from build123d import *
from build123d.topology import SkipClean

# Parameters (mm, degrees)
SKETCH1_W           = 9
SKETCH1_H           = 9
BOSS_EXTRUDE1_DEPTH = 20
SKETCH2_W           = 6
SKETCH2_H           = 6
CUT_EXTRUDE1_DEPTH  = 21.988091862
SKETCH4_W           = 20
SKETCH4_H           = 20
BOSS_EXTRUDE2_DEPTH = 1.5
SKETCH5_W           = 20
SKETCH5_H           = 20
BOSS_EXTRUDE3_DEPTH = 3.5
SKETCH7_W           = 1.8
SKETCH7_H           = 20
CUT_EXTRUDE5_DEPTH  = 16
CUT_EXTRUDE6_START  = -1.7
CUT_EXTRUDE6_DEPTH  = 1.7
BOSS_EXTRUDE4_START = 0.5
BOSS_EXTRUDE4_DEPTH = 0.5
SKETCH10_W          = 6.2
SKETCH10_H          = 6.2
CUT_EXTRUDE8_DEPTH  = 24.748684208


with BuildPart() as part:
    # Sketch1 → Boss-Extrude1 (new body)
    with BuildSketch(Plane.XY):
        Rectangle(SKETCH1_W, SKETCH1_H)
    extrude(amount=BOSS_EXTRUDE1_DEPTH)

    # Sketch2 → Cut-Extrude1 (cut, through all)
    with BuildSketch(Plane(origin=(0, 0, 0), x_dir=(-1, 0, 0), z_dir=(0, 0, -1))):
        Rectangle(SKETCH2_W, SKETCH2_H)
    extrude(amount=-CUT_EXTRUDE1_DEPTH, mode=Mode.SUBTRACT)

    # Sketch4 → Boss-Extrude2 (add)
    with BuildSketch(Plane(origin=(4.5, 0, 0), x_dir=(0, 0, -1), z_dir=(1, 0, 0))):
        with Locations((-10, 0)):
            Rectangle(SKETCH4_W, SKETCH4_H)
    extrude(amount=-BOSS_EXTRUDE2_DEPTH)

    # Sketch5 → Boss-Extrude3 (add)
    with BuildSketch(Plane(origin=(4.5, 0, 0), x_dir=(0, 0, -1), z_dir=(1, 0, 0))):
        with Locations((-10, 0)):
            Rectangle(SKETCH5_W, SKETCH5_H)
    extrude(amount=BOSS_EXTRUDE3_DEPTH)

    # Sketch6 → Cut-Revolve2 (revolve, cut)
    with BuildSketch(Plane(origin=(0, 0, 10), x_dir=(-1, 0, 0), z_dir=(0, 0, -1)), mode=Mode.PRIVATE) as cut_revolve2_sk:
        with BuildLine():
            Line((-4.5, 7.5), (-4.5, 0))
            Line((-4.5, 0), (-7.200284, 0))
            ThreePointArc((-7.200284, 0), (-6.974408022, 3.776920415), (-6.3, 7.5))
            Line((-6.3, 7.5), (-4.5, 7.5))
        make_face()
    revolve(cut_revolve2_sk.sketch.rotate(Axis((88.99, 0, 10), (-1, 0, 0)), 90), axis=Axis((88.99, 0, 10), (-1, 0, 0)), mode=Mode.SUBTRACT)

    # Sketch7 → Cut-Extrude5 (cut)
    with BuildSketch(Plane.XZ.offset(10)):
        with Locations((5.4, 10)):
            Rectangle(SKETCH7_W, SKETCH7_H)
    extrude(amount=-CUT_EXTRUDE5_DEPTH, mode=Mode.SUBTRACT)

    # Sketch8 → Cut-Extrude6 (cut)
    with BuildSketch(Plane(origin=(8, 0, 0), x_dir=(0, 0, -1), z_dir=(1, 0, 0)).offset(CUT_EXTRUDE6_START)):
        with BuildLine():
            Line((-6.875, 0), (-6.875, -10))
            ThreePointArc((-6.875, -10), (-10, -13.125), (-13.125, -10))
            Line((-13.125, -10), (-13.125, 0))
            ThreePointArc((-13.125, 0), (-10, 3.125), (-6.875, 0))
        make_face()
    extrude(amount=CUT_EXTRUDE6_DEPTH, mode=Mode.SUBTRACT)

    # Sketch9 → Boss-Extrude4 (add)
    with SkipClean():  # the faces are left unmerged after this step: merging them gives an invalid solid
        with BuildSketch(Plane.ZY.offset(-6.3).offset(BOSS_EXTRUDE4_START)):
            with BuildLine():
                Line((13.125, -6.817945072), (13.125, -10))
                Line((13.125, -10), (20, -10))
                Line((20, -10), (20, 6))
                Line((20, 6), (14.5, 6))
                ThreePointArc((14.5, 6), (17.457216989, -0.799946739), (13.125, -6.817945072))
            make_face()
            with BuildLine():
                Line((0, -10), (6.875, -10))
                Line((6.875, -10), (6.875, -6.817945072))
                ThreePointArc((6.875, -6.817945072), (2.542783011, -0.799946739), (5.5, 6))
                Line((5.5, 6), (0, 6))
                Line((0, 6), (0, -10))
            make_face()
        extrude(amount=-BOSS_EXTRUDE4_DEPTH)

    # Sketch10 → Cut-Extrude8 (cut, through all)
    with SkipClean():  # the faces are left unmerged after this step: merging them gives an invalid solid
        with BuildSketch(Plane(origin=(0, 0, 0), x_dir=(-1, 0, 0), z_dir=(0, 0, -1))):
            Rectangle(SKETCH10_W, SKETCH10_H)
        extrude(amount=-CUT_EXTRUDE8_DEPTH, mode=Mode.SUBTRACT)


solid = part.part
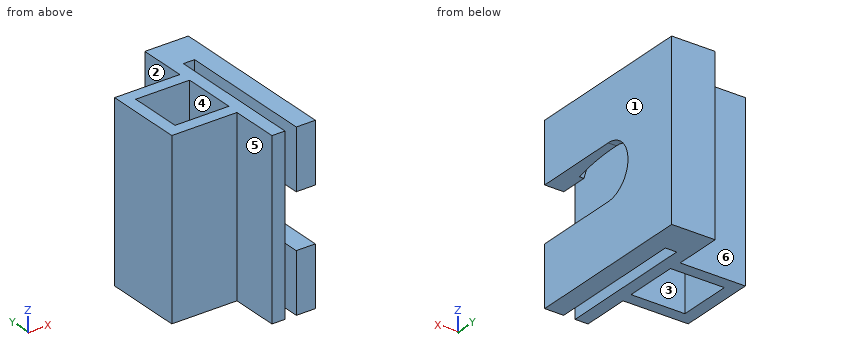
Input: part model. Units: mm. Frame: model coordinates. Face numbers are marked on the shaded views. A direction names the side the tool comes from. Give positions to 0.01 mm unless a question says otherwise; leave off trailing zeros. Loops run counter-clockwise (first coordinate to the right, second up) from the corner with the lowest first, then second, coordinate; pieces in that order, holes last. Notation, with made-up numbers: (89, -11.5) -> (143, -11.5) arc R16 cw to (143, 19.5) -> close; hole circle Ø8 at (54.25, 24.5). An arc over 180 degrees is marked (long way). Answer as a JSON object with one key per item and string values. Group by question number.
Item 1: Cut plane C-C, the plane z = 14. Return the cut outline in (x, y).
Item 2: Cut plane B-B, the plane y = 0.25. Return the cut outline in (x, z), and give its area (3 significant figures).
Item 3: Pull-direction query (X, two-part tool) for the marked faces 1, 2 and 3; classes: released by +X, released by -X, zero draft, split by the parting line, or undercut.
Item 4: Pin query (flat end, axial travel): P1, Ø3, axis at x = -2, z = 14.5, coming from the +Y side; P2, Ø4.5, axis at y = -7.5, z = 6, coming from the -X side; P3, Ø1.9, axis at x = -1, z = 12.5, coming from the -Y side; P4, Ø2, axis at x = 1, y = -8, coming from the +Z side. Return the tip coordinate at first contact, or that it passes through.
Item 5: Cut plane D-D, the plane y = -4.25. Return the cut outline in (x, z) (3 decimals), and give its area (3 significant figures).
Item 6: Reachability of the marked faces 4, 5 and 6 from +Z, -Z, +X, -X, +Y, -Y: full face, straight path, thin tool, end or side. Return the list, or none.
Item 7: Cut plane A-A, the plane x = 1.5. Return the cut outline in (y, z), and give its area (3 significant figures).
Item 8: Line query: probe 1 along X at (y, z) = (-0.5, 14.5); probe 2 along X at (y, z) = (5.25, 3.75); probe 3 along Y at (x, z) = (2.75, 9.25). Output: solid intervals per line, ascending.
Checks:
{
 "1": {"outline": "(-4.5, -4.5) -> (3, -4.5) -> (3, -10) -> (4.5, -10) -> (4.5, 6.34) -> (6.3, 6.34) arc R31.44 cw to (6.3, -6.34) -> (5.8, -6.34) -> (5.8, -10) -> (8, -10) -> (8, 10) -> (3, 10) -> (3, 4.5) -> (-4.5, 4.5) -> close; hole (-3.1, -3.1) -> (3.1, -3.1) -> (3.1, 3.1) -> (-3.1, 3.1) -> close"},
 "2": {"outline": "(-4.5, 0) -> (-3.1, 0) -> (-3.1, 20) -> (-4.5, 20) -> close; (3.1, 0) -> (4.5, 0) -> (4.5, 20) -> (3.1, 20) -> close; (5.8, 0) -> (8, 0) -> (8, 6.89) -> (7.05, 6.89) arc R31.69 cw to (6.3, 2.5) -> (5.8, 2.5) -> close; (5.8, 17.5) -> (6.3, 17.5) arc R31.69 cw to (7.05, 13.11) -> (8, 13.11) -> (8, 20) -> (5.8, 20) -> close", "area": "78.2 mm²"},
 "3": {"face 1": "released by +X", "face 2": "released by -X", "face 3": "undercut"},
 "4": {"P1": "stops at y = 4.5", "P2": "stops at x = 3", "P3": "stops at y = -4.5", "P4": "passes through"},
 "5": {"outline": "(-4.5, 0) -> (4.5, 0) -> (4.5, 20) -> (-4.5, 20) -> close; (5.8, 0) -> (8, 0) -> (8, 6.875) -> (6.758, 6.875) arc R31.404 cw to (6.3, 3.82) -> (5.8, 3.82) -> close; (5.8, 16.18) -> (6.3, 16.18) arc R31.404 cw to (6.758, 13.125) -> (8, 13.125) -> (8, 20) -> (5.8, 20) -> close", "area": "206 mm²"},
 "6": {"face 4": "+Z, -Z", "face 5": "+Z, -Z, -X, -Y", "face 6": "+Z, -Z, -X, +Y"},
 "7": {"outline": "(-4.5, 0) -> (-3.1, 0) -> (-3.1, 20) -> (-4.5, 20) -> close; (3.1, 0) -> (4.5, 0) -> (4.5, 20) -> (3.1, 20) -> close", "area": "56.0 mm²"},
 "8": {"probe 1": "x = -4.5 to -3.1, 3.1 to 4.5, 6.88 to 8", "probe 2": "x = 3 to 4.5, 5.8 to 8", "probe 3": "y = -4.5 to -3.1, 3.1 to 4.5"}
}
